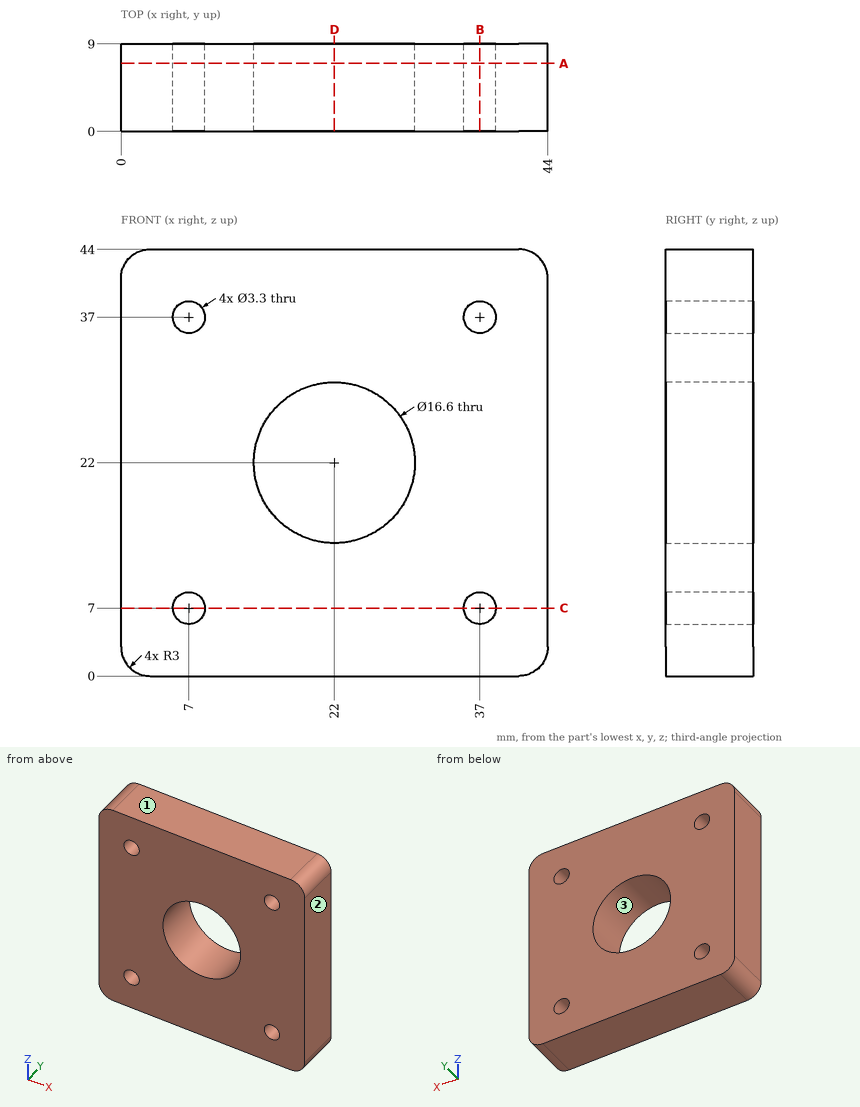
Verification items for this drawing (mm, ordinates from the low corner). Give positions to 0.01 mm unless a question says otherwise; leave off trailing zeros. Write each loop counter-clockwise with the first axis right and the second up, starting at its lowest first coordinate (ties: lowest second). Pieces come first, ordered by that corner, then holes. Notation, with made-up numbers: (-36, -35) - (-12, -35) arc R35 cw to (-12, -2) - close; hole circle Ø6 at (25, -16.75). An arc over 180 degrees is marked (long way). Answer as a JSON object with one key per item and string values. Group by question number.
1) Release check for a two-part mould opening along Z. For the marked faces 1, 2 and 3 record: pulls with the +Z half, pulls with the -Z half, needs draft (parallel to the pull), parting line crosses it, or undercut.
2) Thickness scan on probe 1 along X at (y, z) = (6, 37); probe 2 along X at (y, z) = (4.5, 25.5); probe 3 along X at (y, z) = (4, 29). Record the ranges inside material, lowest first. Write a range as from..to.
3) Sectioned sample at D-D (x = 22). Record the cut outline in (y, z), then the cut area to 3 significant figures.
4) Sectioned sample at C-C (z = 7). Record the cut outline in (x, y).
5) Sectioned sample at A-A (y = 7). Record the cut outline in (x, z).
6) Sectioned sample at B-B (x = 37). Record the cut outline in (y, z), then the cut area to 3 significant figures.
Geometry results:
{
 "1": {"face 1": "pulls with the +Z half", "face 2": "needs draft", "face 3": "undercut"},
 "2": {"probe 1": "x = 0..5.35, 8.65..35.35, 38.65..44", "probe 2": "x = 0..14.47, 29.53..44", "probe 3": "x = 0..17.54, 26.46..44"},
 "3": {"outline": "(0, 0) - (9, 0) - (9, 13.7) - (0, 13.7) - close; (0, 30.3) - (9, 30.3) - (9, 44) - (0, 44) - close", "area": "247 mm^2"},
 "4": {"outline": "(0, 0) - (5.35, 0) - (5.35, 9) - (0, 9) - close; (8.65, 0) - (35.35, 0) - (35.35, 9) - (8.65, 9) - close; (38.65, 0) - (44, 0) - (44, 9) - (38.65, 9) - close"},
 "5": {"outline": "(0, 3) arc R3 ccw to (3, 0) - (41, 0) arc R3 ccw to (44, 3) - (44, 41) arc R3 ccw to (41, 44) - (3, 44) arc R3 ccw to (0, 41) - close; hole circle Ø3.3 at (7, 7); hole circle Ø3.3 at (7, 37); hole circle Ø16.6 at (22, 22); hole circle Ø3.3 at (37, 7); hole circle Ø3.3 at (37, 37)"},
 "6": {"outline": "(0, 0) - (9, 0) - (9, 5.35) - (0, 5.35) - close; (0, 8.65) - (9, 8.65) - (9, 35.35) - (0, 35.35) - close; (0, 38.65) - (9, 38.65) - (9, 44) - (0, 44) - close", "area": "337 mm^2"}
}
